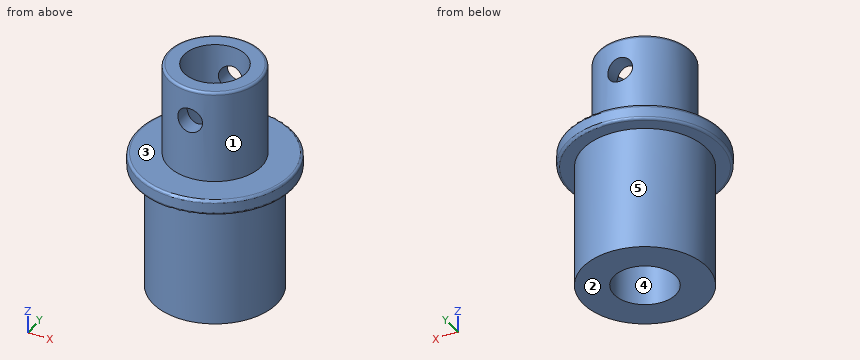
from build123d import *

# Parameters (mm, degrees)
F0_R      = 6.35
F1_DEPTH  = 12.7
F2_R      = 7.9375
F3_DEPTH  = 1.55575
F4_R      = 4.7625
F5_DEPTH  = 9.525
F6_R      = 0.254
F7_R      = 1.27
F8_DEPTH  = 12.7
F9_R      = 3.175
F10_DEPTH = 23.78175


with BuildPart() as f1:
    # F0 (on Top) → F1 (new body)
    with BuildSketch(Plane.XY):
        Circle(F0_R)
    extrude(amount=-F1_DEPTH)

    # F2 (on face) → F3 (join)
    with BuildSketch(Plane.XY):
        Circle(F2_R)
    extrude(amount=F3_DEPTH)

    # F4 (on face) → F5 (join)
    with BuildSketch(Plane.XY.offset(1.55575)):
        Circle(F4_R)
    extrude(amount=F5_DEPTH)

    # F6
    f6_edges = [f1.edges().sort_by_distance(p)[0] for p in [
        (-7.9375, 0, 1.55575),
        (-7.9375, 0, 0),
        (-4.7625, 0, 11.08075),
    ]]
    fillet(f6_edges, radius=F6_R)

    # F7 (on Front) → F8 (cut, symmetric)
    with BuildSketch(Plane.XZ):
        with Locations((0, 7.744468)):
            Circle(F7_R)
    extrude(amount=F8_DEPTH, both=True, mode=Mode.SUBTRACT)

    # F9 (on face) → F10 (cut, through all)
    with BuildSketch(Plane.XY.offset(11.08075)):
        Circle(F9_R)
    extrude(amount=-F10_DEPTH, mode=Mode.SUBTRACT)


solid = f1.part
Check sheet for the modelled part. Datum: model origin and axes. Units: mm. Face numbers are marked on the shaded views. A direction names the side the tool comes from. Round coordinates to 2 decimals unless told otherwise and drop trailing zeros. Order: outer loops, then holes, each group sorted by start corner. A loop starts at its lowest first (then second) coordinate and runs counter-clockwise, first axis right, second up.
(1) Access from +Z, -Z, +X, -X, +Y, -Y to the whole of each face (thin tool, end or side, straight path). Record for the marked faces 1 and 2.
(2) Cross-section at D-D, the plane z = -3.25. Enter the section's corners in (x, y) (3 decimals), and give its area (3 significant figures).
(3) Draft check along X on the marked faces 3, 4 and 5. Enter one of: pulls with the +X half, pulls with the -X half, needs draft (parallel to the pull), parting line crosses it, or undercut.
(4) Cross-section at A-A, the plane x = 0. State how many separate pieces and enclosed holes the cut face has, and give its area (3 significant figures).
(5) Go/stop test with flat-tipped pins: P1, Ø4, axis at x = -2, z = -7, coming from the +Y side; P2, Ø8, axis at x = -6, z = 7.5, coming from the -Y side; P3, Ø5, axis at y = 6.5, z = 3.5, coming from the +X side; P4, Ø4.5, axis at x = 0.5, y = 2.5, coming from the +Z side. Record where each tip stops, or that it passes through.
(6) Scan lines: probe 1 along Z at (x, y) = (0, 4.15); probe 2 along Y at (x, z) = (0, 1.25) (1 decimal); probe 3 along Z at (x, y) = (1.25, -4.75). Record each from-to range of solid material in increasing order.
Check sheet entries:
1. face 1: +Z
1. face 2: -Z, +X, -X, +Y, -Y
2. outline: circle Ø12.7 at (0, 0); hole circle Ø6.35 at (0, 0)
2. area: 95.0 mm2
3. face 3: needs draft
3. face 4: undercut
3. face 5: parting line crosses it
4. separate pieces: 4
4. enclosed holes: 0
4. area: 118 mm2
5. P1: stops at y = 6.35
5. P2: stops at y = -4.32
5. P3: stops at x = 6.05
5. P4: stops at z = 11.08
6. probe 1: z = -12.7 to 6.47, 9.01 to 11.08
6. probe 2: y = -7.9 to -3.2, 3.2 to 7.9
6. probe 3: z = -12.7 to 1.56
